from build123d import *

# Parameters (mm, degrees)
SKETCH1_W           = 203.2
SKETCH1_H           = 101.6
SKETCH1_W_2         = 198.12
SKETCH1_H_2         = 96.52
BOSS_EXTRUDE1_DEPTH = 1526.54
SKETCH2_W           = 99.06
SKETCH2_H           = 609.6
CUT_EXTRUDE1_DEPTH  = 1541.842383763
SKETCH3_W           = 203.2
SKETCH3_H           = 2.54
BOSS_EXTRUDE2_DEPTH = 101.6
CUT_EXTRUDE2_DEPTH  = 1541.928216109


with BuildPart() as part:
    # Sketch1 → Boss-Extrude1 (new body)
    with BuildSketch(Plane(origin=(0, 0, 0), x_dir=(1, 0, 0), z_dir=(0, 1, 0))):
        Rectangle(SKETCH1_W, SKETCH1_H)
        Rectangle(SKETCH1_W_2, SKETCH1_H_2, mode=Mode.SUBTRACT)
    extrude(amount=-BOSS_EXTRUDE1_DEPTH)

    # Sketch2 → Cut-Extrude1 (cut, through all)
    with BuildSketch(Plane(origin=(101.6, 0, 0), x_dir=(0, 0, -1), z_dir=(1, 0, 0))):
        with Locations((-1.27, -1221.74)):
            Rectangle(SKETCH2_W, SKETCH2_H)
    extrude(amount=-CUT_EXTRUDE1_DEPTH, mode=Mode.SUBTRACT)

    # Sketch3 → Boss-Extrude2 (add)
    with BuildSketch(Plane.XY.offset(-48.26)):
        with Locations((0, -1525.27)):
            Rectangle(SKETCH3_W, SKETCH3_H)
    extrude(amount=BOSS_EXTRUDE2_DEPTH)

    # Sketch4 → Cut-Extrude2 (cut, through all)
    with BuildSketch(Plane.ZY.offset(101.6)):
        Polygon((-48.26, -916.94), (-50.8, -916.94), (-50.8, -1526.54), (53.34, -1526.54), (53.34, -1524), (-48.26, -1524), align=None)
    extrude(amount=-CUT_EXTRUDE2_DEPTH, mode=Mode.SUBTRACT)


solid = part.part
For this review, take the finished solid that the model builds, in its own axes (mm). A direction names the side the tool comes from. Give positions to 0.01 mm unless a question says otherwise; leave off trailing zeros. Order: outer loops, then holes, each group sorted by start corner. A loop starts at its lowest first (then second) coordinate and runs counter-clockwise, first axis right, second up. Notation, with made-up numbers: (-38, 34.5) -> (-13, 34.5) arc R21 cw to (-13, 54.5) -> close; hole circle Ø1 at (-32, 71). An arc over 180 degrees is marked (long way). Write item = value, one per line.
1) We need section A-A, the plane x = -75.5. Give the boundary of the cut face in (y, z), and give its area (3 significant figures).
Findings:
outline = (-916.94, -50.8) -> (0, -50.8) -> (0, -48.26) -> (-916.94, -48.26) -> close; (-916.94, 48.26) -> (0, 48.26) -> (0, 50.8) -> (-916.94, 50.8) -> close
area = 4,660 mm^2
2) Draft analysis for pull direction Z (two halves, no side actions). For faces 3 (the face through (1, -465, -48.26)), 4 (the face through (-1, -452, 50.8)), 5 (the face through (0, 0, -49)), state which applies: pulls with the +Z half, pulls with the -Z half, needs draft (parallel to the pull), parting line crosses it, or undercut.
Findings:
face_3 = undercut
face_4 = pulls with the +Z half
face_5 = needs draft
3) For faces 1 (the face through (-1, -452, -50.8)), 2 (the face through (99.06, -452, 1)), list the 3-axis set-ups (+Z, -Z, +X, -X, +Y, -Y) from which the entire face can be reached by the end or side of a thin tool; tool diameter is ignored.
Findings:
face_1 = -Z, +X, -X, +Y, -Y
face_2 = +Y, -Y
4) We need section C-C, the plane y = -637. Give the boundary of the cut face in (x, z), and give its area (3 significant figures).
Findings:
outline = (-101.6, -50.8) -> (101.6, -50.8) -> (101.6, 50.8) -> (-101.6, 50.8) -> close; hole (-99.06, -48.26) -> (99.06, -48.26) -> (99.06, 48.26) -> (-99.06, 48.26) -> close
area = 1,520 mm^2
5) We need section B-B, the plane z = 11. Give the boundary of the cut face in (x, y), and give its area (3 significant figures).
Findings:
outline = (-101.6, -916.94) -> (-99.06, -916.94) -> (-99.06, 0) -> (-101.6, 0) -> close; (99.06, -916.94) -> (101.6, -916.94) -> (101.6, 0) -> (99.06, 0) -> close
area = 4,660 mm^2
6) To check wall thickness, follow L1, parallel to X at y = -135, z = -22; L2, parallel to Z at x = -92.5, y = -679. State the ranges of each line that lie inside material, in increasing order. Write a range as from..to.
Findings:
L1 = -101.6..-99.06, 99.06..101.6
L2 = -50.8..-48.26, 48.26..50.8
